Source: three-view drawing plus pictorial views. Frame: mm from the lowest corner of the part. A direction names the side the tool comes from. Give positions to 0.01 mm unless a question says otherwise; leave off trailing zeros. Loops run counter-clockwise (first coordinate to the right, second up) from the corner with the lowest first, then second, coordinate; pieces in that order, holes last.
1. Access query for the marked faces 1 and 2. Directions: +Z, -Z, +X, -X, +Y, -Y. A direction counts if a zero-diameter tool reaches every point of the face in a straight line with its end or side. Return the directions, or none.
2. Section A-A, the plane z = 1.95. Output: boundary loops of the cut face in (x, y).
3. First-contact query: P1, Ø0.8, axis at y = 5.5, z = 1.5, coming from the +X side; P2, Ø3, axis at x = 32, z = 1.5, coming from the -Y side; P3, Ø1.5, axis at x = 11.5, z = 2.5, coming from the +Y side. Flat tips, straight axial feed; report the tip coordinate or a pass-through.
4. Section B-B, the plane x = 87.5. Output: boundary loops of the cut face in (y, z).
5. Material intervals for line 1 along X through (y, z) = (5.5, 4.7); line 2 along Y through (x, z) = (44.5, 1); line 3 along Y through (x, z) = (74, 3.55), sorted ascending.
6. Draft query along X for the marked faces 3, 4, 5 and 6. Return one class per face: +X half, -X half, draft (parallel to the pull), parting line (faces both ways), or undercut.
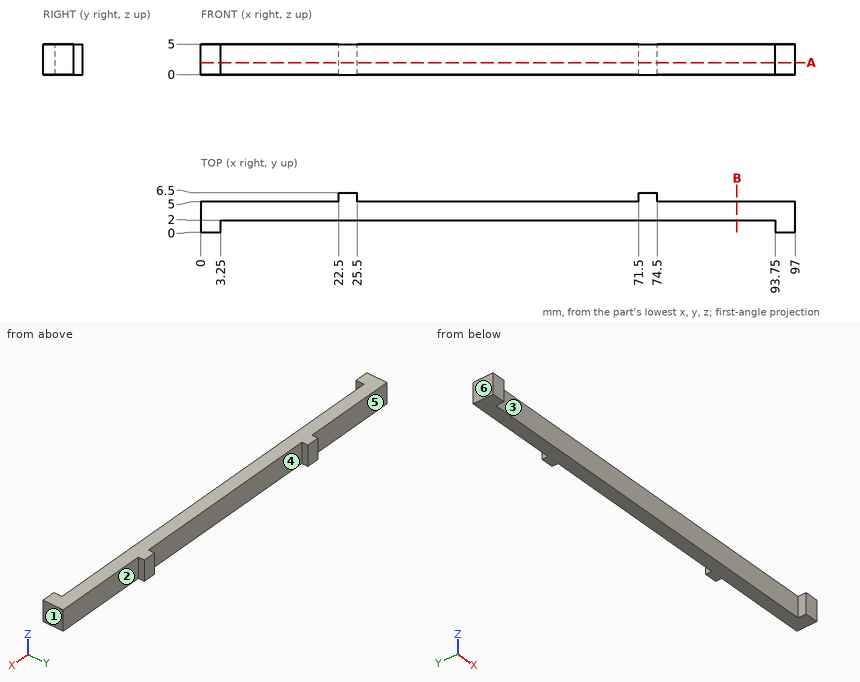
Answers below:
1. face 1: +Z, -Z, +X, +Y, -Y
1. face 2: +Z, -Z, +X, +Y
2. outline: (0, 0) - (3.25, 0) - (3.25, 2) - (93.75, 2) - (93.75, 0) - (97, 0) - (97, 5) - (74.5, 5) - (74.5, 6.5) - (71.5, 6.5) - (71.5, 5) - (25.5, 5) - (25.5, 6.5) - (22.5, 6.5) - (22.5, 5) - (0, 5) - close
3. P1: stops at x = 74.5
3. P2: stops at y = 2
3. P3: stops at y = 5
4. outline: (2, 0) - (5, 0) - (5, 5) - (2, 5) - close
5. line 1: x = 22.5 to 25.5, 71.5 to 74.5
5. line 2: y = 2 to 5
5. line 3: y = 2 to 6.5
6. face 3: undercut
6. face 4: undercut
6. face 5: draft
6. face 6: -X half
